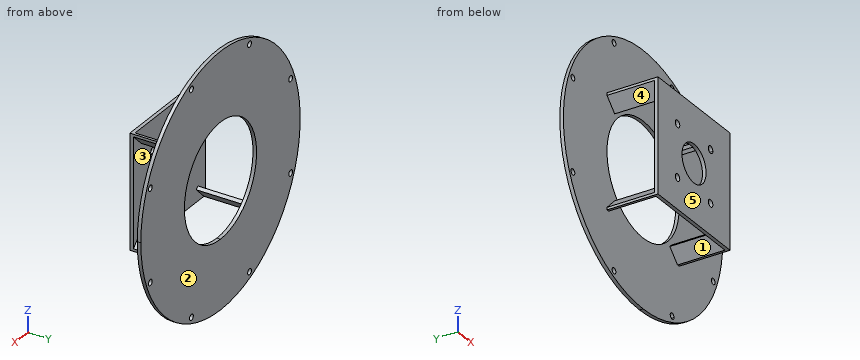
```python
from build123d import *

# Parameters (mm, degrees)
F0_R     = 3.96875
F1_DEPTH = 4.7625
F3_DEPTH = 63.5
F4_R     = 4.7625
F4_R_2   = 25.4
F5_DEPTH = 4.7625


with BuildPart() as f1:
    # F0 (on Front) → F1 (new body)
    with BuildSketch(Plane.XZ):
        with BuildLine():
            ThreePointArc((168.275, 0), (-118.988394, 118.988394), (0, -168.275))
            ThreePointArc((0, -168.275), (32.828824, -165.041643), (64.396055, -155.465828))
            ThreePointArc((64.396055, -155.465828), (139.915549, -93.488581), (168.275, 0))
        make_face()
        with Locations((-61.363365, -148.144268)):
            Circle(F0_R, mode=Mode.SUBTRACT)
        with Locations((-148.144268, -61.363365)):
            Circle(F0_R, mode=Mode.SUBTRACT)
        with BuildLine():
            ThreePointArc((65.332115, -148.144268), (64.66326, -150.349187), (62.88214, -151.810915))
            ThreePointArc((62.88214, -151.810915), (58.06347, -145.939348), (65.332115, -148.144268))
        make_face(mode=Mode.SUBTRACT)
        with Locations((148.144268, -61.363365)):
            Circle(F0_R, mode=Mode.SUBTRACT)
        with Locations((-148.144268, 61.363365)):
            Circle(F0_R, mode=Mode.SUBTRACT)
        with Locations((-61.363365, 148.144268)):
            Circle(F0_R, mode=Mode.SUBTRACT)
        with BuildLine():
            ThreePointArc((152.4, 0), (107.763073, -107.763073), (0, -152.4))
            ThreePointArc((0, -152.4), (-107.763073, 107.763073), (152.4, 0))
        make_face(mode=Mode.SUBTRACT)
        with Locations((148.144268, 61.363365)):
            Circle(F0_R, mode=Mode.SUBTRACT)
        with Locations((61.363365, 148.144268)):
            Circle(F0_R, mode=Mode.SUBTRACT)
        with BuildLine():
            ThreePointArc((152.4, 0), (-107.763073, 107.763073), (0, -152.4))
            ThreePointArc((0, -152.4), (107.763073, -107.763073), (152.4, 0))
        make_face()
        with BuildLine():
            ThreePointArc((0, -76.2), (-53.881537, 53.881537), (76.2, 0))
            ThreePointArc((76.2, 0), (53.881537, -53.881537), (0, -76.2))
        make_face(mode=Mode.SUBTRACT)
    extrude(amount=F1_DEPTH)

    # F2 (on face) → F3 (join)
    with BuildSketch(Plane.XZ.offset(4.7625)):
        Polygon((-56.55569, 59.923286), (-72.832404, 76.2), (-76.2, 76.2), (-76.2, 72.832404), (-59.923286, 56.55569), (-58.239488, 58.239488), align=None)
        Polygon((59.923286, 56.55569), (76.2, 72.832404), (76.2, 76.2), (72.832404, 76.2), (56.55569, 59.923286), (58.239488, 58.239488), align=None)
        Polygon((76.2, -76.2), (76.2, -72.832404), (59.923286, -56.55569), (58.239488, -58.239488), (56.55569, -59.923286), (72.832404, -76.2), align=None)
        Polygon((-76.2, -76.2), (-72.832404, -76.2), (-56.55569, -59.923286), (-58.239488, -58.239488), (-59.923286, -56.55569), (-76.2, -72.832404), align=None)
    extrude(amount=F3_DEPTH)

    # F4 (on face) → F5 (join)
    with BuildSketch(Plane.XZ.offset(68.2625)):
        Polygon((-72.832404, 76.2), (-76.2, 76.2), (-76.2, -76.2), (76.2, -76.2), (76.2, 76.2), align=None)
        with Locations((-34.925, -34.925)):
            Circle(F4_R, mode=Mode.SUBTRACT)
        with Locations((34.925, -34.925)):
            Circle(F4_R, mode=Mode.SUBTRACT)
        with Locations((-34.925, 34.925)):
            Circle(F4_R, mode=Mode.SUBTRACT)
        Circle(F4_R_2, mode=Mode.SUBTRACT)
        with BuildLine():
            ThreePointArc((39.6875, 34.925), (38.292596, 31.557404), (34.925, 30.1625))
            ThreePointArc((34.925, 30.1625), (31.557404, 38.292596), (39.6875, 34.925))
        make_face(mode=Mode.SUBTRACT)
    extrude(amount=F5_DEPTH)


solid = f1.part
```
Can you work these out from the model? Positions are in its coordinate system, mm. Face numbers are marked on the shaded views. A direction names the side the tool comes from. Give positions to 0.01 mm unless a question says otherwise; leave off trailing zeros. Loops run counter-clockwise (first coordinate to the right, second up) from the corner with the lowest first, then second, coordinate; pieces in that order, holes last. Notation, with made-up numbers: M -32,25 L -17,25 A29 ccw -17,63 Z; hole C 9.25,24 d7. An arc over 180 degrees is marked long. Use CSV: the item, a comma, the result in double quotes. Start each with the question number.
1. Imagine slicing it at B-B, the plane x = -86. Write out the boundary of the cut face in (y, z).
2. On a 3-axis mill with a long thin cutter (end or side, diameter ignored), from which of +Z, -Z, +X, -X, +Y, -Y can I reach the whole of each face in a straight line? I mean the marked faces 1 and 2. Say none if no direction works.
3. If we mould it in two halves opening along X, with no side actions, what happens to the marked faces 3, 4 and 5? For each: released by +X, released by -X, zero draft, split by the parting line, or undercut.
4. If I drill on L1, parallel to Y at x = -31, z = 143.5; L2, parallel to Y at x = -54, z = 31.5 (1 decimal); L3, parallel to Z at x = 64, y = -24, over which ranges is the centre line in solid material (lowest first)?
5. Imagine slicing it at C-C, the plane z = -100.5. Write out the boundary of the cut face in (x, y).
6. For P1, Ø8, axis at x = -122, z = 1.5, coming from the -Y side; P2, Ø7, axis at x = -61.36, z = 148.14, coming from the +Y side; P3, Ø10, axis at x = 61, z = 108.5, coming from the +Y side; P4, Ø6, axis at y = -27.5, z = 58.5, coming from the -X side, each with a flat end and sliding along its axis, tell me the tip position at first contact or that it passes through.
7. Imagine slicing it at A-A, the plane y = -50.5. Write out the boundary of the cut face in (x, z), plus the area to 3 significant figures.
Response values:
1,outline,"M -4.76,-144.64 L 0,-144.64 L 0,144.64 L -4.76,144.64 Z"
2,face 1,"-Z"
2,face 2,"+Z, -Z, +X, -X, +Y"
3,face 3,"undercut"
3,face 4,"released by -X"
3,face 5,"zero draft"
4,L1,"-4.76 to 0"
4,L2,"-73 to -68.3"
4,L3,"-67.37 to -60.63, 60.63 to 67.37"
5,outline,"M -134.97,-4.76 L 134.97,-4.76 L 134.97,0 L -134.97,0 Z"
6,P1,"y = -4.76"
6,P2,"through"
6,P3,"y = 0"
6,P4,"x = -64.87"
7,outline,"M -76.2,-76.2 L -72.83,-76.2 L -56.56,-59.92 L -59.92,-56.56 L -76.2,-72.83 Z; M -76.2,72.83 L -59.92,56.56 L -56.56,59.92 L -72.83,76.2 L -76.2,76.2 Z; M 56.56,-59.92 L 72.83,-76.2 L 76.2,-76.2 L 76.2,-72.83 L 59.92,-56.56 Z; M 56.56,59.92 L 59.92,56.56 L 76.2,72.83 L 76.2,76.2 L 72.83,76.2 Z"
7,area,"461 mm^2"
